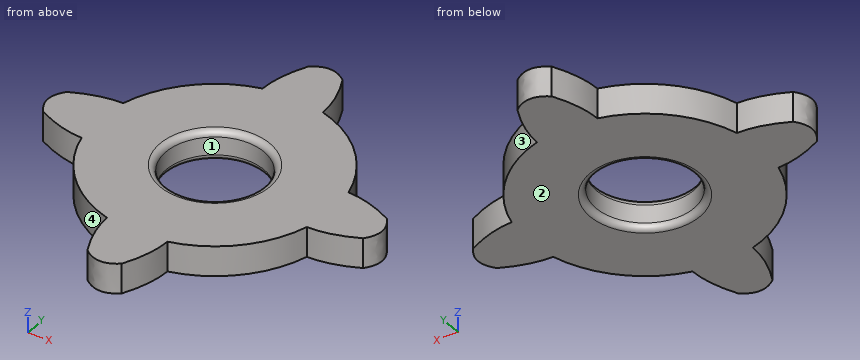
from build123d import *

# Parameters (mm, degrees)
SKETCH1_R           = 16.342033632
BOSS_EXTRUDE1_DEPTH = 10
FILLET1_R           = 2
FILLET2_R           = 2


with BuildPart() as part:
    # Sketch1 → Boss-Extrude1 (new body)
    with BuildSketch(Plane.XY):
        with BuildLine():
            ThreePointArc((-37.630023744, -10.082934473), (-27.54708927, -27.54708927), (-10.082934473, -37.630023744))
            add(Edge.make_bspline(
                [(-5.730379822, -53.435114302), (-9.976997746, -45.009715936), (-10.082934473, -37.630023744)],
                knots=[0, 0, 0, 1, 1, 1], degree=2))
            add(Edge.make_bspline(
                [(5.730379822, -53.435114302), (0, -58.17853574), (-5.730379822, -53.435114302)],
                knots=[0, 0, 0, 1, 1, 1], degree=2))
            add(Edge.make_bspline(
                [(5.730379822, -53.435114302), (9.976997746, -45.009715936), (10.082934473, -37.630023744)],
                knots=[0, 0, 0, 1, 1, 1], degree=2))
            ThreePointArc((10.082934473, -37.630023744), (27.54708927, -27.54708927), (37.630023744, -10.082934473))
            add(Edge.make_bspline(
                [(53.435114302, -5.730379822), (45.009715936, -9.976997746), (37.630023744, -10.082934473)],
                knots=[0, 0, 0, 1, 1, 1], degree=2))
            add(Edge.make_bspline(
                [(53.435114302, 5.730379822), (58.17853574, 0), (53.435114302, -5.730379822)],
                knots=[0, 0, 0, 1, 1, 1], degree=2))
            add(Edge.make_bspline(
                [(53.435114302, 5.730379822), (45.009715936, 9.976997746), (37.630023744, 10.082934473)],
                knots=[0, 0, 0, 1, 1, 1], degree=2))
            ThreePointArc((37.630023744, 10.082934473), (27.54708927, 27.54708927), (10.082934473, 37.630023744))
            add(Edge.make_bspline(
                [(5.730379822, 53.435114302), (9.976997746, 45.009715936), (10.082934473, 37.630023744)],
                knots=[0, 0, 0, 1, 1, 1], degree=2))
            add(Edge.make_bspline(
                [(-5.730379822, 53.435114302), (0, 58.17853574), (5.730379822, 53.435114302)],
                knots=[0, 0, 0, 1, 1, 1], degree=2))
            add(Edge.make_bspline(
                [(-5.730379822, 53.435114302), (-9.976997746, 45.009715936), (-10.082934473, 37.630023744)],
                knots=[0, 0, 0, 1, 1, 1], degree=2))
            ThreePointArc((-10.082934473, 37.630023744), (-27.54708927, 27.54708927), (-37.630023744, 10.082934473))
            add(Edge.make_bspline(
                [(-53.435114302, 5.730379822), (-45.009715936, 9.976997746), (-37.630023744, 10.082934473)],
                knots=[0, 0, 0, 1, 1, 1], degree=2))
            add(Edge.make_bspline(
                [(-53.435114302, -5.730379822), (-58.17853574, 0), (-53.435114302, 5.730379822)],
                knots=[0, 0, 0, 1, 1, 1], degree=2))
            add(Edge.make_bspline(
                [(-53.435114302, -5.730379822), (-45.009715936, -9.976997746), (-37.630023744, -10.082934473)],
                knots=[0, 0, 0, 1, 1, 1], degree=2))
        make_face()
        Circle(SKETCH1_R, mode=Mode.SUBTRACT)
    extrude(amount=BOSS_EXTRUDE1_DEPTH)

    # Fillet1
    fillet1_edges = [part.edges().sort_by_distance(p)[0] for p in [
        (-16.342033632, 0, 0),
    ]]
    fillet(fillet1_edges, radius=FILLET1_R)

    # Fillet2
    fillet2_edges = [part.edges().sort_by_distance(p)[0] for p in [
        (-16.342033632, 0, 10),
    ]]
    fillet(fillet2_edges, radius=FILLET2_R)


solid = part.part
The model under review builds one solid part; all positions refer to its coordinate system, in mm. Face numbers are marked on the shaded views. Round coordinates to 2 decimals unless told otherwise and drop trailing zeros. Order: outer loops, then holes, each group sorted by start corner. A loop starts at its lowest first (then second) coordinate and runs counter-clockwise, first axis right, second up. Notation, with made-up numbers: (59, -29.75) -> (85, -29.75) arc R9 cw to (85, -22.75) -> close; hole circle Ø8 at (88, 80.5). An arc over 180 degrees is marked (long way). Return JSON: item names as keys, results as strings.
1. Insertion check: P1, Ø3, axis at x = -19.5, z = 7.5, coming from the +Y side; P2, Ø5, axis at x = -33, y = 1, coming from the -Z side; P3, Ø1.5, axis at x = -16, z = 4, coming from the -Y side; P4, Ø2, axis at x = -12, y = -43, coming from the +Z side. Each pin has a flat end and moves straight along its axis. Give the tip position at first contact, or say it passes through.
Answer block:
{"P1": "stops at y = 34.55", "P2": "stops at z = 0", "P3": "stops at y = -35.85", "P4": "passes through"}
2. Take a section at B-B (y = 35). Write out the cut boundary in (x, z), then the cut area to 3 significant figures.
Answer block:
{"outline": "(-17.11, 0) -> (17.11, 0) -> (17.11, 10) -> (-17.11, 10) -> close", "area": "342 mm²"}
3. The part is to be moulded in two halves that separate along Y. For the marked faces 1, 2, 3 and 4, say which applies: +Y half, -Y half, draft (parallel to the pull), parting line (faces both ways), or undercut.
Answer block:
{"face 1": "undercut", "face 2": "draft", "face 3": "+Y half", "face 4": "-Y half"}
4. Take a section at A-A (x = 27.5). Write out the cut boundary in (y, z), then the cut area to 3 significant figures.
Answer block:
{"outline": "(-27.59, 0) -> (27.59, 0) -> (27.59, 10) -> (-27.59, 10) -> close", "area": "552 mm²"}
5. For L1, parallel to Y at x = 0, z = 3.6; L2, parallel to X at y = 7, z = 9.25; L3, parallel to X at y = 12.5, z = 7, list the stretches that pass through material, from the lowest coordinate up. Write a range as [from, to].
Answer block:
{"L1": "y = [-55.81, -16.34], [16.34, 55.81]", "L2": "x = [-50.73, -15.25], [15.25, 50.73]", "L3": "x = [-36.9, -10.53], [10.53, 36.9]"}
